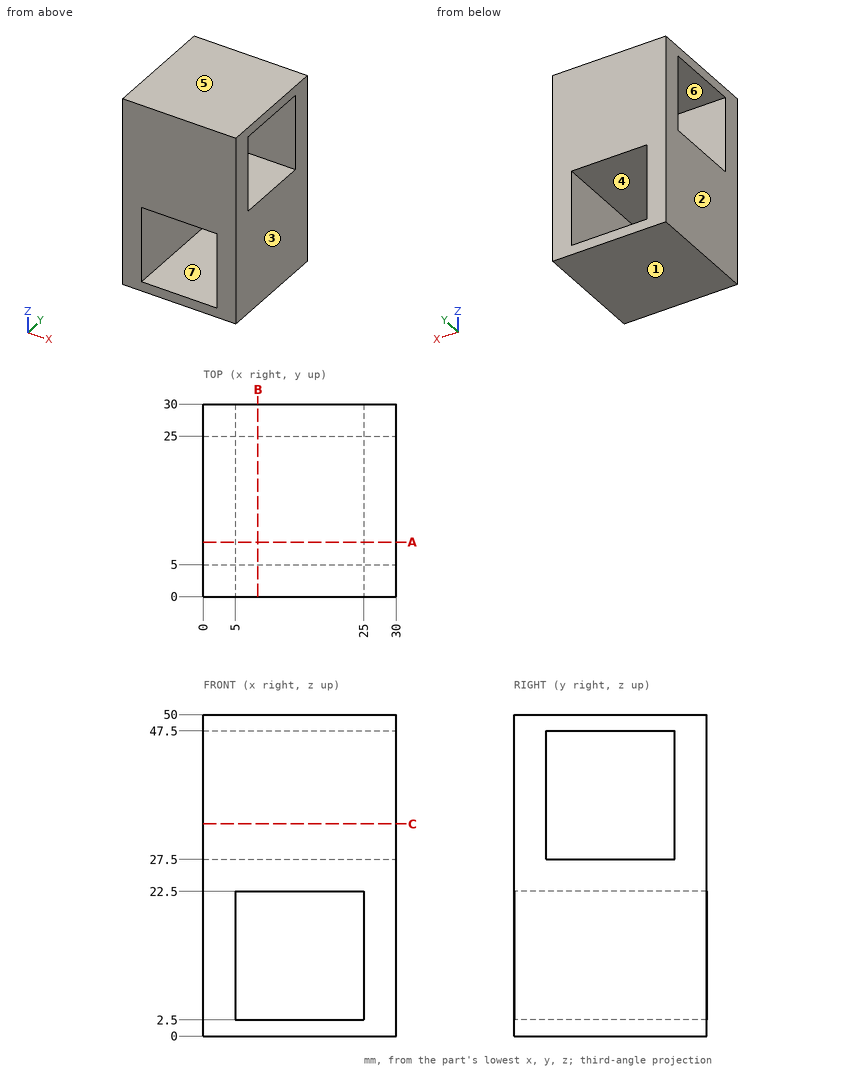
Check sheet for the drawn part. Datum: minimum x, y, z corner. Units: mm. A direction names the side the tool comes from. Round coordinates to 2 decimals unless told otherwise and drop trailing zeros. Write each loop counter-clockwise with the first axis right and the second up, starting at its lowest first coordinate (ties: lowest second). Pieces come first, ordered by that corner, then holes. Notation, with made-up numbers: (-3, 27) - (40, 27) arc R18 cw to (40, 32) - close; hole circle Ø3 at (72, 10). An arc over 180 degrees is marked (long way). Return JSON: item names as keys, results as strings.
Q1. Depth check by flat-ended pin: P1, Ø16, axis at x = 7.5, z = 38.5, coming from the -Y side. Enter the tip coordinate at first touch or a pass-through.
Returned:
{"P1": "stops at y = 0"}
Q2. Scan lines: L1, parallel to Z at x = 12.25, y = 23.25; L2, parallel to Y at x = 2.5, z = 33.5. Record each from-to range of solid material in increasing order. Write a range as from..to.
Returned:
{"L1": "z = 0..2.5, 22.5..27.5, 47.5..50", "L2": "y = 0..5, 25..30"}
Q3. Cross-section at C-C (z = 33). Record the boundary of the cut face in (x, y).
Returned:
{"outline": "(0, 0) - (30, 0) - (30, 5) - (0, 5) - close; (0, 25) - (30, 25) - (30, 30) - (0, 30) - close"}
Q4. Cross-section at A-A (y = 8.5). Record the boundary of the cut face in (x, z).
Returned:
{"outline": "(0, 0) - (30, 0) - (30, 27.5) - (0, 27.5) - close; (0, 47.5) - (30, 47.5) - (30, 50) - (0, 50) - close; hole (5, 2.5) - (25, 2.5) - (25, 22.5) - (5, 22.5) - close"}
Q5. Draft check along X on the marked faces 1, 2, 3 and 4. Enter one of: released by +X, released by -X, zero draft, split by the parting line, or undercut.
Returned:
{"face 1": "zero draft", "face 2": "released by -X", "face 3": "released by +X", "face 4": "undercut"}
Q6. Cross-section at B-B (x = 8.5). Record the boundary of the cut face in (y, z), then the cut area to 3 significant figures.
Returned:
{"outline": "(0, 0) - (30, 0) - (30, 2.5) - (0, 2.5) - close; (0, 22.5) - (30, 22.5) - (30, 50) - (0, 50) - close; hole (5, 27.5) - (25, 27.5) - (25, 47.5) - (5, 47.5) - close", "area": "500 mm²"}
Q7. Access from +Z, -Z, +X, -X, +Y, -Y to the whole of each face (thin tool, end or side, straight path). Record for the marked faces 5, 6 and 7.
Returned:
{"face 5": "+Z, +X, -X, +Y, -Y", "face 6": "+X, -X", "face 7": "+Y, -Y"}
